from build123d import *

# Parameters (mm, degrees)
SKETCH1_W                  = 12.7
SKETCH1_H                  = 76.2
BOSS_EXTRUDE1_DEPTH        = 25.4
F_97_0_31_DIAMETER_HOLE1_D = 7.874
FILLET1_R                  = 2.54


with BuildPart() as part:
    # Sketch1 → Boss-Extrude1 (new body)
    with BuildSketch(Plane.XY):
        Rectangle(SKETCH1_W, SKETCH1_H)
    extrude(amount=BOSS_EXTRUDE1_DEPTH)

    # #97 (0.31) Diameter Hole1 (through all)
    with Locations(Plane(origin=(6.35, 0, 0), x_dir=(0, 0, -1), z_dir=(1, 0, 0))):
        with Locations((-12.7, 25.4), (-12.7, -25.4)):
            Hole(F_97_0_31_DIAMETER_HOLE1_D / 2)

    # Fillet1
    fillet1_edges = [part.edges().sort_by_distance(p)[0] for p in [
        (-6.35, 0, 25.4),
        (0, -38.1, 25.4),
        (6.35, 0, 25.4),
        (0, -38.1, 0),
        (-6.35, 0, 0),
        (0, 38.1, 0),
        (6.35, 0, 0),
        (6.35, -38.1, 12.7),
        (-6.35, -38.1, 12.7),
        (-6.35, 38.1, 12.7),
        (6.35, 38.1, 12.7),
        (0, 38.1, 25.4),
    ]]
    fillet(fillet1_edges, radius=FILLET1_R)


solid = part.part
For this review, take the finished solid that the model builds, in its own axes (mm). Coordinates: 2 decimals unless noted, no trailing zeros. Loops run counter-clockwise (first coordinate to the right, second up) from the corner with the lowest first, then second, coordinate; pieces in that order, holes last. Notation, with made-up numbers: (88, 12.5) - (120, 12.5) arc R12 cw to (120, 29.5) - close; hole circle Ø1 at (73.25, 26.5). An arc over 180 degrees is marked (long way). Return JSON: item names as keys, results as strings.
Item 1: Take a section at A-A (z = 12.7). Give the boundary of the cut face in (x, y), then the cut area to 3 significant figures.
Determined:
{"outline": "(-6.35, -35.56) arc R2.54 ccw to (-3.81, -38.1) - (3.81, -38.1) arc R2.54 ccw to (6.35, -35.56) - (6.35, -29.34) - (-6.35, -29.34) - close; (-6.35, -21.46) - (6.35, -21.46) - (6.35, 21.46) - (-6.35, 21.46) - close; (-6.35, 29.34) - (6.35, 29.34) - (6.35, 35.56) arc R2.54 ccw to (3.81, 38.1) - (-3.81, 38.1) arc R2.54 ccw to (-6.35, 35.56) - close", "area": "762 mm2"}
Item 2: Mouldability with a two-part tool opening along X and no side actions: class faces 1 (the cylindrical face through (-5.626, 0.498, 0.764)), 2 (the cylindrical face through (0.053, -37.376, 0.764)), 3 (the cylindrical face through (5.586, -37.376, 12.842)) as pulls with the +X half, pulls with the -X half, needs draft (parallel to the pull), parting line crosses it, or undercut.
Determined:
{"face 1": "pulls with the -X half", "face 2": "needs draft", "face 3": "pulls with the +X half"}
Item 3: Take a section at D-D (y = 12). Give the boundary of the cut face in (x, z), then the cut area to 3 significant figures.
Determined:
{"outline": "(-6.35, 2.54) arc R2.54 ccw to (-3.81, 0) - (3.81, 0) arc R2.54 ccw to (6.35, 2.54) - (6.35, 22.86) arc R2.54 ccw to (3.81, 25.4) - (-3.81, 25.4) arc R2.54 ccw to (-6.35, 22.86) - close", "area": "317 mm2"}
Item 4: Take a section at B-B (x = 1.25). Give the boundary of the cut face in (y, z), then the cut area to 3 significant figures.
Determined:
{"outline": "(-38.1, 2.54) arc R2.54 ccw to (-35.56, 0) - (35.56, 0) arc R2.54 ccw to (38.1, 2.54) - (38.1, 22.86) arc R2.54 ccw to (35.56, 25.4) - (-35.56, 25.4) arc R2.54 ccw to (-38.1, 22.86) - close; hole circle Ø7.87 at (-25.4, 12.7); hole circle Ø7.87 at (25.4, 12.7)", "area": "1,830 mm2"}
Item 5: Take a section at C-C (y = 25.4). Give the boundary of the cut face in (x, z).
Determined:
{"outline": "(-6.35, 2.54) arc R2.54 ccw to (-3.81, 0) - (3.81, 0) arc R2.54 ccw to (6.35, 2.54) - (6.35, 8.76) - (-6.35, 8.76) - close; (-6.35, 16.64) - (6.35, 16.64) - (6.35, 22.86) arc R2.54 ccw to (3.81, 25.4) - (-3.81, 25.4) arc R2.54 ccw to (-6.35, 22.86) - close"}
Item 6: For line 1 (Y direction, x = -3, z = 12.7); line 2 (Y direction, x = -4.5, z = 13); line 3 (Z direction, x = -1, y = 27), list the stretches that pass through material, from the lowest coordinate up.
Determined:
{"line 1": "y = -38.1 to -29.34, -21.46 to 21.46, 29.34 to 38.1", "line 2": "y = -38 to -29.33, -21.47 to 21.47, 29.33 to 38", "line 3": "z = 0 to 9.1, 16.3 to 25.4"}
